Design review of the part built by this model. Coordinates are the model's own, in mm. A direction names the side the tool comes from. Coordinates: 2 decimals unless noted, no trailing zeros. Write each loop counter-clockwise with the first axis right and the second up, starting at its lowest first coordinate (ties: lowest second). Pieces come first, ordered by that corner, then holes.
Q1. The part is to be moulded in two halves that separate along X. For faces 4 (the flat face through (10, 23, 10)), 5 (the flat face through (-20, 16, 10)), 6 (the flat face through (8.7, 27, 11.3)), 7 (the cylindrical face through (9.1, 25, 8.8)), say which applies: released by +X, released by -X, zero draft, split by the parting line, or undercut.
Q2. Take a section at B-B, the plane x = 1.5. Write out the cut boundary in (y, z), plus the area to 3 significant figures.
Q3. Take a section at C-C, the plane y = 22. Write out the cut boundary in (x, z), plus the area to 3 significant figures.
Q4. For L1, parallel to X at y = 24, z = 10; L2, parallel to X at y = -2, z = 7; L3, parallel to Y at x = 13.5, z = 10, list the stretches that pass through material, from the lowest coordinate up.
Q5. Take a section at D-D, the plane x = 23. Write out the cut boundary in (y, z).
Q6. For pin 1 Ø6 at (y, z) = (-0.5, 3.5) entering from -X; pin 2 Ø2 at (y, z) = (6, 7) entering from +X; pin 3 Ø3.5 at (x, z) = (-24, 5.5) entering from +Y; pin 4 Ø8 at (x, y) = (-8.5, 15.5) entering from -Z, all flat-tipped, find the tip position at first contact; note any pin that passes through.
Q7. Take a section at A-A, the plane z = 10. Write out the cut boundary in (x, y).
Q8. For faces 1 (the cylindrical face through (19, 21, 10)), 2 (the flat face through (-9, 20, 3)), 3 (the flat face through (-0.35, 21.48, 2.48)), list the 3-axis set-ups (+Z, -Z, +X, -X, +Y, -Y) from which the entire face can be reached by the end or side of a thin tool; tool diameter is ignored.
from build123d import *

# Parameters (mm, degrees)
SKETCH_1_W      = 40
SKETCH_1_H      = 40
EXTRUDE_1_DEPTH = 20
EXTRUDE_2_DEPTH = 3
SKETCH_5_R      = 3
SKETCH_5_R_2    = 1.5
EXTRUDE_3_DEPTH = 4
SKETCH_6_W      = 7
SKETCH_6_H      = 2
EXTRUDE_4_DEPTH = 20


with BuildPart() as part:
    # 草图1 → 凸台-拉伸1 (new body)
    with BuildSketch(Plane.XY):
        Rectangle(SKETCH_1_W, SKETCH_1_H)
    extrude(amount=EXTRUDE_1_DEPTH)

    # 草图2 → 凸台-拉伸2 (add)
    with BuildSketch(Plane(origin=(0, 20, 0), x_dir=(1, 0, 0), z_dir=(0, 1, 0))):
        with BuildLine():
            Line((10, -1), (-11, -4))
            ThreePointArc((-11, -4), (-16.99824603, -9.854932566), (-11.290050053, -15.992985147))
            Line((-11.290050053, -15.992985147), (10, -19))
            ThreePointArc((10, -19), (19, -10), (10, -1))
        make_face()
    extrude(amount=EXTRUDE_2_DEPTH)

    # 草图5 → 凸台-拉伸3 (add)
    with BuildSketch(Plane(origin=(0, 23, 0), x_dir=(1, 0, 0), z_dir=(0, 1, 0))):
        with Locations(Location((10, -10, 0), (0, 0, 270))):
            Circle(SKETCH_5_R)
        with Locations(Location((10, -10, 0), (0, 0, 270))):
            Circle(SKETCH_5_R_2, mode=Mode.SUBTRACT)
    extrude(amount=EXTRUDE_3_DEPTH)

    # 草图6 → 凸台-拉伸4 (add)
    with BuildSketch(Plane(origin=(0, 0, 0), x_dir=(-1, 0, 0), z_dir=(0, 0, -1))):
        with Locations((-23.5, 12)):
            Rectangle(SKETCH_6_W, SKETCH_6_H)
        with Locations((23.5, 12)):
            Rectangle(SKETCH_6_W, SKETCH_6_H)
    extrude(amount=-EXTRUDE_4_DEPTH)


solid = part.part
Responses:
1. face 4: undercut
1. face 5: released by -X
1. face 6: zero draft
1. face 7: undercut
2. outline: (-20, 0) - (20, 0) - (20, 2.21) - (23, 2.21) - (23, 17.8) - (20, 17.8) - (20, 20) - (-20, 20) - close
2. area: 847 mm2
3. outline: (-11.29, 15.99) arc R6 ccw to (-11, 4) - (10, 1) arc R9 ccw to (10, 19) - close
3. area: 499 mm2
4. L1: x = 7 to 8.5, 11.5 to 13
4. L2: x = -20 to 20
4. L3: y = -20 to 23
5. outline: (11, 0) - (13, 0) - (13, 20) - (11, 20) - close
6. pin 1: stops at x = -20
6. pin 2: stops at x = 20
6. pin 3: stops at y = 13
6. pin 4: stops at z = 0
7. outline: (-27, 11) - (-20, 11) - (-20, -20) - (20, -20) - (20, 11) - (27, 11) - (27, 13) - (20, 13) - (20, 20) - (19, 20) - (19, 23) - (13, 23) - (13, 27) - (11.5, 27) - (11.5, 23) - (8.5, 23) - (8.5, 27) - (7, 27) - (7, 23) - (-17, 23) - (-17, 20) - (-20, 20) - (-20, 13) - (-27, 13) - close
8. face 1: +X, +Y
8. face 2: +Y
8. face 3: -Z, -X, +Y
